```python
from build123d import *

# Parameters (mm, degrees)
SKETCH1_W           = 60
SKETCH1_H           = 50
SKETCH1_R           = 1
BOSS_EXTRUDE1_DEPTH = 1.6


with BuildPart() as part:
    # Sketch1 → Boss-Extrude1 (new body)
    with BuildSketch(Plane.XY):
        with Locations((2.183616654, 0.548157273)):
            Rectangle(SKETCH1_W, SKETCH1_H)
        with Locations((-22.816383346, 20.548157273)):
            Circle(SKETCH1_R, mode=Mode.SUBTRACT)
        with Locations(Location((27.183616654, 20.548157273, 0), (0, 0, 180))):
            Circle(SKETCH1_R, mode=Mode.SUBTRACT)
        with Locations((27.183616654, -19.451842727)):
            Circle(SKETCH1_R, mode=Mode.SUBTRACT)
        with Locations(Location((-22.816383346, -19.451842727, 0), (0, 0, 180))):
            Circle(SKETCH1_R, mode=Mode.SUBTRACT)
        with BuildLine():
            Line((-0.849639296, -12.726842727), (5.150360704, -12.726842727))
            Line((5.150360704, -12.726842727), (5.150360704, -16.19097143))
            ThreePointArc((5.150360704, -16.19097143), (17.594007322, -6.629576314), (16.906048518, 9.048157273))
            Line((16.906048518, 9.048157273), (16.040023114, 8.548157273))
            ThreePointArc((16.040023114, 8.548157273), (2.183616654, 16.548157273), (-11.672789807, 8.548157273))
            Line((-11.672789807, 8.548157273), (-12.538815211, 9.048157273))
            ThreePointArc((-12.538815211, 9.048157273), (-13.241008775, -6.598935169), (-0.849639296, -16.179046867))
            Line((-0.849639296, -16.179046867), (-0.849639296, -12.726842727))
        make_face(mode=Mode.SUBTRACT)
    extrude(amount=BOSS_EXTRUDE1_DEPTH)


solid = part.part
```
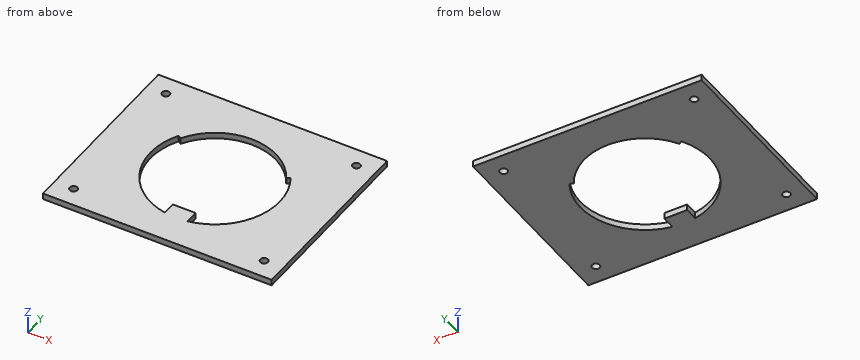
The model under review builds one solid part; all positions refer to its coordinate system, in mm. Coordinates: 2 decimals unless noted, no trailing zeros. Order: outer loops, then holes, each group sorted by start corner. A loop starts at its lowest first (then second) coordinate and runs counter-clockwise, first axis right, second up. Notation, with made-up numbers: (6.5, 18) -> (19.5, 18) arc R18 cw to (19.5, 45) -> close; hole circle Ø1 at (28, 9.25). An arc over 180 degrees is marked (long way). Answer in a Markdown table with one row per item. Add a question column.
Item 1: We need section C-C on z = 1.1. Write out the cut boundary in (x, y).
Item 2: We need section B-B on y = -5. Write out the cut boundary in (x, z), plus the area to 3 significant figures.
Item 3: We need section A-A on x = -3. Write out the cut boundary in (y, z).
Item 4: To check wall thickness, follow probe 1 along X at (y, z) = (-13, 1.1); probe 2 along Y at (x, z) = (27, 0.85); probe 3 along X at (y, z) = (0, 0.75). State the ranges of each line that lie inside material, in increasing order.
Final values:
| question | item | result |
|---|---|---|
| 1 | outline | (-27.82, -24.45) -> (32.18, -24.45) -> (32.18, 25.55) -> (-27.82, 25.55) -> close; hole circle Ø2 at (-22.82, -19.45); hole circle Ø2 at (-22.82, 20.55); hole (-12.54, 9.05) arc R17 ccw to (-0.85, -16.18) -> (-0.85, -12.73) -> (5.15, -12.73) -> (5.15, -16.19) arc R17 ccw to (16.91, 9.05) -> (16.04, 8.55) arc R16 ccw to (-11.67, 8.55) -> close; hole circle Ø2 at (27.18, -19.45); hole circle Ø2 at (27.18, 20.55) |
| 2 | outline | (-27.82, 0) -> (-13.89, 0) -> (-13.89, 1.6) -> (-27.82, 1.6) -> close; (18.25, 0) -> (32.18, 0) -> (32.18, 1.6) -> (18.25, 1.6) -> close |
| 2 | area | 44.6 mm2 |
| 3 | outline | (-24.45, 0) -> (-15.64, 0) -> (-15.64, 1.6) -> (-24.45, 1.6) -> close; (15.69, 0) -> (25.55, 0) -> (25.55, 1.6) -> (15.69, 1.6) -> close |
| 4 | probe 1 | x = -27.82 to -8.09, -0.85 to 5.15, 12.45 to 32.18 |
| 4 | probe 2 | y = -24.45 to -20.43, -18.47 to 19.57, 21.53 to 25.55 |
| 4 | probe 3 | x = -27.82 to -14.81, 19.17 to 32.18 |
